Here's how the part is built. I have some questions about the finished solid (model axes, mm). A direction names the side the tool comes from. Coordinates: 2 decimals unless noted, no trailing zeros. Order: outer loops, then holes, each group sorted by start corner. A loop starts at its lowest first (then second) coordinate and runs counter-clockwise, first axis right, second up. Notation, with made-up numbers: (87, 79) - (138, 79) arc R14 cw to (138, 95) - close; hole circle Ø5 at (23, -8.5). An arc over 180 degrees is marked (long way). Use CSV: the item, a comma, the result in double quotes. Start each with the question number.
from build123d import *

# Parameters (mm, degrees)
SKETCH1_W           = 70
SKETCH1_H           = 35
BOSS_EXTRUDE1_DEPTH = 32
SKETCH2_R           = 4
CUT_EXTRUDE1_DEPTH  = 59.940648113
CHAMFER1_SIZE       = 25
SKETCH3_W           = 44
SKETCH3_H           = 7
BOSS_EXTRUDE2_DEPTH = 47
FILLET1_R           = 10
FILLET2_R           = 10
SKETCH4_W           = 3
SKETCH4_H           = 63
BOSS_EXTRUDE3_DEPTH = 47
FILLET3_R           = 2


with BuildPart() as part:
    # Sketch1 → Boss-Extrude1 (new body)
    with BuildSketch(Plane(origin=(0, 0, 0), x_dir=(1, 0, 0), z_dir=(0, 1, 0))):
        Rectangle(SKETCH1_W, SKETCH1_H)
    extrude(amount=BOSS_EXTRUDE1_DEPTH)

    # Sketch2 → Cut-Extrude1 (cut, through all)
    with BuildSketch(Plane.XY.offset(17.5)):
        with Locations((0, 25)):
            Circle(SKETCH2_R)
    extrude(amount=-CUT_EXTRUDE1_DEPTH, mode=Mode.SUBTRACT)

    # Chamfer1
    chamfer1_edges = [part.edges().sort_by_distance(p)[0] for p in [
        (-35, 32, 0),
        (35, 32, 0),
    ]]
    chamfer(chamfer1_edges, length=CHAMFER1_SIZE)

    # Sketch3 → Boss-Extrude2 (add)
    with BuildSketch(Plane(origin=(35, 0, 0), x_dir=(0, 0, -1), z_dir=(1, 0, 0))):
        with Locations((0, 3.5)):
            Rectangle(SKETCH3_W, SKETCH3_H)
    extrude(amount=BOSS_EXTRUDE2_DEPTH)

    # Fillet1
    # the kernel refuses this fillet: 10 mm, written as the material it adds along each edge
    with BuildSketch(Plane(origin=(35, 0, -17.5), x_dir=(-1.5347723092402642e-12, 0, -1.0), z_dir=(0, 1, 0))) as fillet1_piece_1_section:
        with BuildLine():
            CenterArc((10, 8.351646544), FILLET1_R, 180, 56.632987031)
            Line((0, 8.351646544), (-0.2, 8.351646544))
            Line((-0.2, 8.351646544), (-0.2, 0))
            Line((-0.2, 0), (0, -0.2))
            ThreePointArc((0, -0.2), (2.25, -0.2), (4.39, -0.167032931))
            Line((4.39, -0.167032931), (4.5, 0))
        make_face()
    fillet1_piece_1 = extrude(amount=7, mode=Mode.PRIVATE)
    fillet1_piece_1 = split(fillet1_piece_1, bisect_by=Plane(origin=(35.692594852, 6.307405148, -18.660307251), z_dir=(-0.7071067811865476, -0.7071067811865476, 0)), keep=Keep.TOP, mode=Mode.PRIVATE)
    add(fillet1_piece_1)
    with BuildSketch(Plane(origin=(35, 0, -17.5), x_dir=(-1.5347723092402642e-12, 0, -1.0), z_dir=(0, 1, 0))) as fillet1_piece_2_section:
        with BuildLine():
            CenterArc((10, 8.351646544), FILLET1_R, 180, 56.632987031)
            Line((0, 8.351646544), (-0.2, 8.351646544))
            Line((-0.2, 8.351646544), (-0.2, 0))
            Line((-0.2, 0), (0, -0.2))
            ThreePointArc((0, -0.2), (2.25, -0.2), (4.39, -0.167032931))
            Line((4.39, -0.167032931), (4.5, 0))
        make_face()
    fillet1_piece_2 = extrude(amount=27.879116361, mode=Mode.PRIVATE)
    fillet1_piece_2 = split(fillet1_piece_2, bisect_by=Plane(origin=(31.191797934, 7, -18.092333784), z_dir=(0, 1, 0)), keep=Keep.TOP, mode=Mode.PRIVATE)
    fillet1_piece_2 = split(fillet1_piece_2, bisect_by=Plane(origin=(32.143848451, 9.856151549, -18.092333784), z_dir=(-0.7071067811865476, -0.7071067811865476, 0)), keep=Keep.TOP, mode=Mode.PRIVATE)
    add(fillet1_piece_2)
    with BuildSketch(Plane(origin=(35, 0, -17.5), x_dir=(-1.5347723092402642e-12, 0, -1.0), z_dir=(0, 1, 0))) as fillet1_piece_3_section:
        with BuildLine():
            CenterArc((10, 8.351646544), FILLET1_R, 180, 56.632987031)
            Line((0, 8.351646544), (-0.2, 8.351646544))
            Line((-0.2, 8.351646544), (-0.2, 0))
            Line((-0.2, 0), (0, -0.2))
            ThreePointArc((0, -0.2), (2.25, -0.2), (4.39, -0.167032931))
            Line((4.39, -0.167032931), (4.5, 0))
        make_face()
    fillet1_piece_3 = extrude(amount=7, mode=Mode.PRIVATE)
    fillet1_piece_3 = split(fillet1_piece_3, bisect_by=Plane(origin=(35.097400014, 6.902599986, -19.555271065), z_dir=(0.7071067811865476, 0.7071067811865476, 0)), keep=Keep.TOP, mode=Mode.PRIVATE)
    add(fillet1_piece_3)

    # Fillet2
    # the kernel refuses this fillet: 10 mm, written as the material it adds along each edge
    with BuildSketch(Plane(origin=(35, 0, 17.5), x_dir=(-1.5331933253830236e-12, 0, 1.0), z_dir=(0, 1, 0))) as fillet2_piece_1_section:
        with BuildLine():
            CenterArc((10, -8.351646544), FILLET2_R, 123.367012969, 56.632987031)
            Line((0, -8.351646544), (-0.2, -8.351646544))
            Line((-0.2, -8.351646544), (-0.2, 0))
            Line((-0.2, 0), (0, 0.2))
            ThreePointArc((0, 0.2), (2.25, 0.2), (4.39, 0.167032931))
            Line((4.39, 0.167032931), (4.5, 0))
        make_face()
    fillet2_piece_1 = extrude(amount=7, mode=Mode.PRIVATE)
    fillet2_piece_1 = split(fillet2_piece_1, bisect_by=Plane(origin=(35.692594852, 6.307405148, 18.660307251), z_dir=(-0.7071067811865476, -0.7071067811865476, 0)), keep=Keep.TOP, mode=Mode.PRIVATE)
    add(fillet2_piece_1)
    with BuildSketch(Plane(origin=(35, 0, 17.5), x_dir=(-1.5331933253830236e-12, 0, 1.0), z_dir=(0, 1, 0))) as fillet2_piece_2_section:
        with BuildLine():
            CenterArc((10, -8.351646544), FILLET2_R, 123.367012969, 56.632987031)
            Line((0, -8.351646544), (-0.2, -8.351646544))
            Line((-0.2, -8.351646544), (-0.2, 0))
            Line((-0.2, 0), (0, 0.2))
            ThreePointArc((0, 0.2), (2.25, 0.2), (4.39, 0.167032931))
            Line((4.39, 0.167032931), (4.5, 0))
        make_face()
    fillet2_piece_2 = extrude(amount=27.879116361, mode=Mode.PRIVATE)
    fillet2_piece_2 = split(fillet2_piece_2, bisect_by=Plane(origin=(31.191797934, 7, 18.092333784), z_dir=(0, 1, 0)), keep=Keep.TOP, mode=Mode.PRIVATE)
    fillet2_piece_2 = split(fillet2_piece_2, bisect_by=Plane(origin=(32.143848451, 9.856151549, 18.092333784), z_dir=(-0.7071067811865476, -0.7071067811865476, 0)), keep=Keep.TOP, mode=Mode.PRIVATE)
    add(fillet2_piece_2)
    with BuildSketch(Plane(origin=(35, 0, 17.5), x_dir=(-1.5331933253830236e-12, 0, 1.0), z_dir=(0, 1, 0))) as fillet2_piece_3_section:
        with BuildLine():
            CenterArc((10, -8.351646544), FILLET2_R, 123.367012969, 56.632987031)
            Line((0, -8.351646544), (-0.2, -8.351646544))
            Line((-0.2, -8.351646544), (-0.2, 0))
            Line((-0.2, 0), (0, 0.2))
            ThreePointArc((0, 0.2), (2.25, 0.2), (4.39, 0.167032931))
            Line((4.39, 0.167032931), (4.5, 0))
        make_face()
    fillet2_piece_3 = extrude(amount=7, mode=Mode.PRIVATE)
    fillet2_piece_3 = split(fillet2_piece_3, bisect_by=Plane(origin=(35.097400014, 6.902599986, 19.555271065), z_dir=(0.7071067811865476, 0.7071067811865476, 0)), keep=Keep.TOP, mode=Mode.PRIVATE)
    add(fillet2_piece_3)

    # Sketch4 → Boss-Extrude3 (add)
    with BuildSketch(Plane(origin=(0, 7, 0), x_dir=(1, 0, 0), z_dir=(0, 1, 0))):
        with Locations((80.5, 0)):
            Rectangle(SKETCH4_W, SKETCH4_H)
    extrude(amount=BOSS_EXTRUDE3_DEPTH)

    # Fillet3
    fillet3_edges = [part.edges().sort_by_distance(p)[0] for p in [
        (80.5, 7, 22),
        (80.5, 7, -22),
        (82, 0, 0),
        (80.5, 7, -31.5),
        (80.5, 7, 31.5),
    ]]
    fillet(fillet3_edges, radius=FILLET3_R)


solid = part.part
Item 1: We'd pull the mould along Y, two halves only. Please class faces 1 (the flat face through (58, 3, -22)), 2 (the flat face through (23, 19, 0)), 3 (the cylindrical face through (-0.521, 28.966, 0.245)): released by +Y, released by -Y, zero draft, split by the parting line, or undercut.
Item 2: Please list where these lines run through material, in increasing order: line 1 along Y through (x, z) = (0, -3); line 2 along X through (y, z) = (12.5, 0); line 3 along X through (y, z) = (28, -9). Write a range as from..to.
Item 3: Suppose I cut it at A-A on y = 25. Write out the boundary of the cut face in (x, z), then the cut area to 3 significant figures.
Item 4: Suppose I cut it at B-B on x = 0. Write out the boundary of the cut face in (y, z), then the cut area to 3 significant figures.
Item 5: For faces 4 (the flat face through (-5, 12, -17.5)), 5 (the flat face through (80, 7, -27)), 6 (the flat face through (79, 29, 0)), which set-ups out of +Z, -Z, +X, -X, +Y, -Y let a thin tool reach every point of the face, with its end or its side?
Item 6: Suppose I cut it at C-C on z = 10. Write out the boundary of the cut face in (x, y).
Item 7: Suppose I cut it at D-D on y = 11.5. Write out the boundary of the cut face in (x, z), then the cut area to 3 significant figures.
Item 8: For pin 1 Ø2 at (y, z) = (44, -1.5) entering from -X; pin 2 Ø13 at (x, y) = (0, 25) entering from +Z; pin 3 Ø1.5 at (x, z) = (15, 20) entering from -Y; pin 4 Ø7.5 at (x, y) = (56, 3.5) entering from +Z, each with a flat end and sliding along its axis, tell me the tip position at first contact or that it passes through.
Here are the results:
1,face 1,"zero draft"
1,face 2,"released by +Y"
1,face 3,"undercut"
2,line 1,"0..21, 29..32"
2,line 2,"-29.5..29.5, 79..82"
2,line 3,"-14..-2.65, 2.65..14, 79..82"
3,outline,"(-17, -17.5) - (-4, -17.5) - (-4, 17.5) - (-17, 17.5) - close; (4, -17.5) - (17, -17.5) - (17, 17.5) - (4, 17.5) - close; (79, -31.5) - (82, -31.5) - (82, 31.5) - (79, 31.5) - close"
3,area,"1,100 mm^2"
4,outline,"(0, -17.5) - (21, -17.5) - (21, 17.5) - (0, 17.5) - close; (29, -17.5) - (32, -17.5) - (32, 17.5) - (29, 17.5) - close"
4,area,"840 mm^2"
5,face 4,"-Z, -X, +Y, -Y"
5,face 5,"-Z, +X, -X, -Y"
5,face 6,"+Z, -Z, +Y"
6,outline,"(-35, 0) - (80, 0) arc R2 ccw to (82, 2) - (82, 54) - (79, 54) - (79, 7) - (35, 7) - (10, 32) - (-10, 32) - (-35, 7) - close; hole circle Ø8 at (0, 25)"
7,outline,"(-30.5, -17.5) - (26.65, -17.5) arc R10 cw to (30.5, -18.27) - (30.5, 18.27) arc R10 cw to (26.65, 17.5) - (-30.5, 17.5) - close; (79, -31.5) - (82, -31.5) - (82, 31.5) - (79, 31.5) - close"
7,area,"2,330 mm^2"
8,pin 1,"x = 79"
8,pin 2,"z = 17.5"
8,pin 3,"through"
8,pin 4,"z = 22"
